Source: CAD feature listing. Evaluate the final solid. Frame: model axes, mm. Face numbers are marked on the shaded views. A direction names the side the tool comes from. Coordinates: 2 decimals unless noted, no trailing zeros. Order: outer loops, then holes, each group sorted by start corner. A loop starts at its lowest first (then second) coordinate and runs counter-clockwise, first axis right, second up. Notation, with made-up numbers: (52.5, 48.25) -> (60.5, 48.25) arc R20 ccw to (60.5, 76.25) -> close; hole circle Ø1 at (18.25, -15.75). An arc over 180 degrees is marked (long way). Put each result on its own line as item: value.
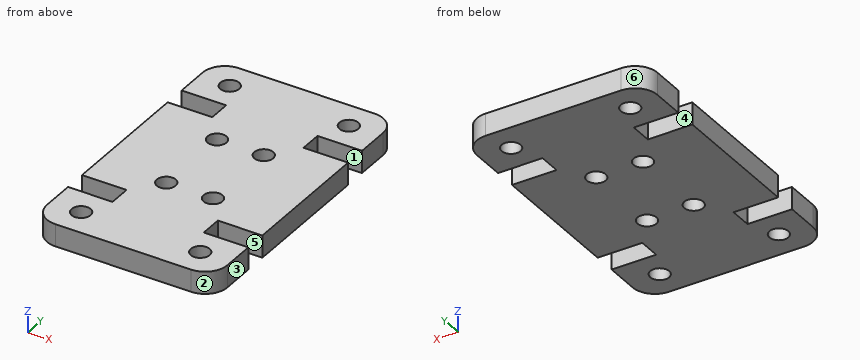
from build123d import *

# Parameters (mm, degrees)
SKETCH2_R           = 0.85
BOSS_EXTRUDE1_DEPTH = 4
SKETCH3_W           = 16.2
SKETCH3_H           = 26.26
CUT_EXTRUDE1_DEPTH  = 2


with BuildPart() as part:
    # Sketch2 → Boss-Extrude1 (new body)
    with BuildSketch(Plane.XY):
        with BuildLine():
            Line((0, 7), (0, 19.26))
            Line((0, 19.26), (4, 19.26))
            Line((4, 19.26), (4, 21.26))
            Line((4, 21.26), (0, 21.26))
            Line((0, 21.26), (0, 24.26))
            ThreePointArc((0, 24.26), (0.585786438, 25.674213562), (2, 26.26))
            Line((2, 26.26), (14.2, 26.26))
            ThreePointArc((14.2, 26.26), (15.614213562, 25.674213562), (16.2, 24.26))
            Line((16.2, 24.26), (16.2, 21.26))
            Line((16.2, 21.26), (12.2, 21.26))
            Line((12.2, 21.26), (12.2, 19.26))
            Line((12.2, 19.26), (16.2, 19.26))
            Line((16.2, 19.26), (16.2, 7))
            Line((16.2, 7), (12.2, 7))
            Line((12.2, 7), (12.2, 5))
            Line((12.2, 5), (16.2, 5))
            Line((16.2, 5), (16.2, 2))
            ThreePointArc((16.2, 2), (15.614213562, 0.585786438), (14.2, 0))
            Line((14.2, 0), (2, 0))
            ThreePointArc((2, 0), (0.585786438, 0.585786438), (0, 2))
            Line((0, 2), (0, 5))
            Line((0, 5), (4, 5))
            Line((4, 5), (4, 7))
            Line((4, 7), (0, 7))
        make_face()
        with Locations((13.45, 2.5)):
            Circle(SKETCH2_R, mode=Mode.SUBTRACT)
        with Locations((10.2, 9.5)):
            Circle(SKETCH2_R, mode=Mode.SUBTRACT)
        with Locations((2.75, 23.76)):
            Circle(SKETCH2_R, mode=Mode.SUBTRACT)
        with Locations((6, 16.76)):
            Circle(SKETCH2_R, mode=Mode.SUBTRACT)
        with Locations((10.2, 16.76)):
            Circle(SKETCH2_R, mode=Mode.SUBTRACT)
        with Locations((13.45, 23.76)):
            Circle(SKETCH2_R, mode=Mode.SUBTRACT)
        with Locations((6, 9.5)):
            Circle(SKETCH2_R, mode=Mode.SUBTRACT)
        with Locations((2.75, 2.5)):
            Circle(SKETCH2_R, mode=Mode.SUBTRACT)
    extrude(amount=BOSS_EXTRUDE1_DEPTH)

    # Sketch3 → Cut-Extrude1 (cut)
    with BuildSketch(Plane.XY.offset(4)):
        with Locations((8.1, 13.13)):
            Rectangle(SKETCH3_W, SKETCH3_H)
    extrude(amount=-CUT_EXTRUDE1_DEPTH, mode=Mode.SUBTRACT)


solid = part.part
1. Cut plane B-B on y = 16.76. Output: boundary loops of the cut face in (x, z).
Numbers:
outline: (0, 0) -> (5.15, 0) -> (5.15, 2) -> (0, 2) -> close; (6.85, 0) -> (9.35, 0) -> (9.35, 2) -> (6.85, 2) -> close; (11.05, 0) -> (16.2, 0) -> (16.2, 2) -> (11.05, 2) -> close
2. Cut plane C-C on x = 13.45. Output: boundary loops of the cut face in (y, z).
Numbers:
outline: (0, 0) -> (1.65, 0) -> (1.65, 2) -> (0, 2) -> close; (3.35, 0) -> (5, 0) -> (5, 2) -> (3.35, 2) -> close; (7, 0) -> (19.26, 0) -> (19.26, 2) -> (7, 2) -> close; (21.26, 0) -> (22.91, 0) -> (22.91, 2) -> (21.26, 2) -> close; (24.61, 0) -> (26.26, 0) -> (26.26, 2) -> (24.61, 2) -> close
3. Cut plane A-A on x = 6. Output: boundary loops of the cut face in (y, z), plus the area to 3 significant figures.
Numbers:
outline: (0, 0) -> (8.65, 0) -> (8.65, 2) -> (0, 2) -> close; (10.35, 0) -> (15.91, 0) -> (15.91, 2) -> (10.35, 2) -> close; (17.61, 0) -> (26.26, 0) -> (26.26, 2) -> (17.61, 2) -> close
area: 45.7 mm2
4. Pull-direction query (Y, two-part tool) for the marked faces 1, 2 and 3; classes: pulls with the +Y half, pulls with the -Y half, needs draft (parallel to the pull), parting line crosses it, or undercut.
Numbers:
face 1: undercut
face 2: pulls with the -Y half
face 3: needs draft
5. Set-up query: the marked faces 4, 5 and 6. Return all of +Z, -Z, +X, -X, +Y, -Y with unobstructed straight access to the full face (end or side cutting, diameter ignored); none if empty.
Numbers:
face 4: +Z, -Z, -X
face 5: +Z, -Z, +X
face 6: +Z, -Z, -X, +Y
6. Ray query, line 1 along X through (y, z) = (16.76, 0.45); line 2 along Y through (x, z) = (12.5, 1.5); line 3 along Y through (x, z) = (13.45, 1.3). Return the intervals inside material, ascending.
Numbers:
line 1: x = 0 to 5.15, 6.85 to 9.35, 11.05 to 16.2
line 2: y = 0 to 5, 7 to 19.26, 21.26 to 26.26
line 3: y = 0 to 1.65, 3.35 to 5, 7 to 19.26, 21.26 to 22.91, 24.61 to 26.26
7. First-contact query: pin 1 (1.4 mm diameter, centred on x = 2.75, y = 2.5, fed in from +Z); pin 2 (0.6 mm diameter, centred on x = 1, z = 1, fed in from +Y). Flat tips, straight axial feed; report the tip coordinate or a pass-through.
Numbers:
pin 1: passes through
pin 2: stops at y = 26.13
8. Cut plane D-D on z = 0.35. Count the separate pieces of the cut face and the enclosed holes in it, plus the area to 3 significant figures.
Numbers:
separate pieces: 1
enclosed holes: 8
area: 372 mm2
